Part model, mm, in its own coordinate system. A direction names the side the tool comes from. Give positions to 0.01 mm unless a question says otherwise; leave off trailing zeros. Write each loop counter-clockwise with the first axis right and the second up, starting at its lowest first coordinate (ties: lowest second). Pieces come first, ordered by that corner, then holes.
```python
from build123d import *

# Parameters (mm, degrees)
BOSS_EXTRU_4_DEPTH = 5


with BuildPart() as part:
    # Esquisse1 → Boss.-Extru.4 (new body)
    with BuildSketch(Plane.XY):
        Polygon((-275.915909498, -82.850341845), (-268.915909498, -82.850341845), (-268.915909498, -81.850341845), (-265.915909498, -81.850341845), (-265.915909498, -82.850341845), (-235.915909498, -82.850341845), (-235.915909498, -81.850341845), (-232.915909498, -81.850341845), (-232.915909498, -82.850341845), (-225.915909498, -82.850341845), (-210.915909498, -56.869579731), (-210.915909498, -49.869579731), (-211.915909498, -49.869579731), (-211.915909498, -46.869579731), (-210.915909498, -46.869579731), (-210.915909498, -16.869579731), (-211.915909498, -16.869579731), (-211.915909498, -13.869579731), (-210.915909498, -13.869579731), (-210.915909498, -6.869579731), (-225.915909498, 19.111182382), (-232.915909498, 19.111182382), (-232.915909498, 18.111182382), (-235.915909498, 18.111182382), (-235.915909498, 19.111182382), (-265.915909498, 19.111182382), (-265.915909498, 18.111182382), (-268.915909498, 18.111182382), (-268.915909498, 19.111182382), (-275.915909498, 19.111182382), (-290.915909498, -6.869579731), (-290.915909498, -13.869579731), (-289.915909498, -13.869579731), (-289.915909498, -16.869579731), (-290.915909498, -16.869579731), (-290.915909498, -46.869579731), (-289.915909498, -46.869579731), (-289.915909498, -49.869579731), (-290.915909498, -49.869579731), (-290.915909498, -56.869579731), align=None)
        Polygon((-283.915909498, -49.869579731), (-283.915909498, -54.993935384), (-260.915909498, -31.869817618), (-283.915909498, -8.745224078), (-283.915909498, -13.869579731), (-284.915909498, -13.869579731), (-284.915909498, -16.869579731), (-283.915909498, -16.869579731), (-283.915909498, -46.869579731), (-284.915909498, -46.869579731), (-284.915909498, -49.869579731), align=None, mode=Mode.SUBTRACT)
        Polygon((-268.915909498, 12.111182382), (-271.874457613, 12.111182382), (-250.915909498, -21.869817618), (-229.957361382, 12.111182382), (-232.915909498, 12.111182382), (-232.915909498, 13.111182382), (-235.915909498, 13.111182382), (-235.915909498, 12.111182382), (-265.915909498, 12.111182382), (-265.915909498, 13.111182382), (-268.915909498, 13.111182382), align=None, mode=Mode.SUBTRACT)
        Polygon((-271.874457613, -75.850341845), (-250.915909498, -41.869817618), (-229.957361382, -75.850341845), (-232.915909498, -75.850341845), (-232.915909498, -76.850341845), (-235.915909498, -76.850341845), (-235.915909498, -75.850341845), (-265.915909498, -75.850341845), (-265.915909498, -76.850341845), (-268.915909498, -76.850341845), (-268.915909498, -75.850341845), align=None, mode=Mode.SUBTRACT)
        Polygon((-217.915909498, -54.993935384), (-240.915909498, -31.869817618), (-217.915909498, -8.745224078), (-217.915909498, -13.869579731), (-216.915909498, -13.869579731), (-216.915909498, -16.869579731), (-217.915909498, -16.869579731), (-217.915909498, -46.869579731), (-216.915909498, -46.869579731), (-216.915909498, -49.869579731), (-217.915909498, -49.869579731), align=None, mode=Mode.SUBTRACT)
    extrude(amount=BOSS_EXTRU_4_DEPTH)


solid = part.part
```
1) Saw through at B-B, the plane y = 7. Write the cut outline in (x, z), then the cut area to 3 significant figures.
Answers follow:
outline: (-282.91, 0) - (-268.72, 0) - (-268.72, 5) - (-282.91, 5) - close; (-233.11, 0) - (-218.92, 0) - (-218.92, 5) - (-233.11, 5) - close
area: 142 mm2
2) Wall check: L1, parallel to Y at x = -237, z = 4.2; L2, parallel to X at y = -29, z = 2.1; L3, parallel to Y at x = -254.5, z = 1.7. Give the ranges that are in metal, low to high.
Answers follow:
L1: y = -82.85 to -75.85, -64.43 to -35.81, -27.93 to 0.69, 12.11 to 19.11
L2: x = -290.92 to -283.92, -263.77 to -238.06, -217.92 to -210.92
L3: y = -82.85 to -75.85, -47.68 to -16.06, 12.11 to 19.11
3) Pin check, flat tips, straight feed: pin 1 Ø2.5 at (y, z) = (-15.5, 3) entering from -X; pin 2 Ø6 at (x, y) = (-238, -35.5) entering from -Z; pin 3 Ø1.5 at (x, z) = (-234, 2) entering from -Y; pin 4 Ø0.8 at (y, z) = (12.5, 1.5) entering from -X. Stop position of each tip, or through.
Answers follow:
pin 1: stops at x = -289.92
pin 2: stops at z = 0
pin 3: stops at y = -81.85
pin 4: stops at x = -279.96
4) Saw through at D-D, the plane z = 1.45. Count the separate pieces of the cut face and the enclosed holes in it, then the cut area to 3 significant figures.
Answers follow:
separate pieces: 1
enclosed holes: 4
area: 4,840 mm2
5) Saw through at A-A, the plane x = -282. Write the cut outline in (y, z), then the cut area to 3 significant figures.
Answers follow:
outline: (-72.31, 0) - (-53.07, 0) - (-53.07, 5) - (-72.31, 5) - close; (-10.67, 0) - (8.57, 0) - (8.57, 5) - (-10.67, 5) - close
area: 192 mm2
6) 3-axis set-ups, long thin cutter, end or side, ignore diameter. For faces 5 (the face through (-234, -81.85, 2)), 6 (the face through (-218.31, 5.94, 2.46)), 7 (the face through (-283.916, -32, 2)), 8 (the face through (-211.916, -15, 2)), 9 (the face through (-272, -82.85, 2)): which of +Z, -Z, +X, -X, +Y, -Y reach the whole face in a straight line?
Answers follow:
face 5: +Z, -Z, -Y
face 6: +Z, -Z, +X, +Y
face 7: +Z, -Z
face 8: +Z, -Z, +X
face 9: +Z, -Z, +X, -X, -Y
7) Two-plate mould, pull along Y, no slides. Class faces 1 (the face through (-210.916, -53, 2)), 2 (the face through (-261.542, -4.641, 2.465)), 3 (the face through (-272, 19.111, 2)), 4 (the face through (-283.52, -69.68, 2.46)): +Y half, -Y half, draft (parallel to the pull), parting line (faces both ways), or undercut.
Answers follow:
face 1: draft
face 2: undercut
face 3: +Y half
face 4: -Y half
8) Saw through at C-C, the plane x = -248. Write the cut outline in (y, z).
Answers follow:
outline: (-82.85, 0) - (-75.85, 0) - (-75.85, 5) - (-82.85, 5) - close; (-46.6, 0) - (-17.14, 0) - (-17.14, 5) - (-46.6, 5) - close; (12.11, 0) - (19.11, 0) - (19.11, 5) - (12.11, 5) - close
